```python
from build123d import *

# Parameters (mm, degrees)
ESQUISSE1_R                                   = 7
BOSS_EXTRU_1_DEPTH                            = 60
ESQUISSE3_R                                   = 7.5
BOSS_EXTRU_2_DEPTH                            = 62
ESQUISSE4_R                                   = 7.5
BOSS_EXTRU_3_DEPTH                            = 12
ESQUISSE5_R                                   = 7
BOSS_EXTRU_4_DEPTH                            = 26
ENL_V_MAT_EXTRU_1_DEPTH                       = 2.96
ENL_V_MAT_EXTRU_2_DEPTH                       = 2.96
TROU_POUR_TARAUDAGE_POUR_TROU_TARAUD_M6_D     = 5
TROU_POUR_TARAUDAGE_POUR_TROU_TARAUD_M6_DEPTH = 15
TROU_POUR_TARAUDAGE_POUR_TROU_TARAUD_M6_TIP   = 1.502151548
TROU_POUR_TARAUDAGE_POUR_TROU_TARAUD_2_D      = 5
TROU_POUR_TARAUDAGE_POUR_TROU_TARAUD_2_DEPTH  = 15
TROU_POUR_TARAUDAGE_POUR_TROU_TARAUD_2_TIP    = 1.502151548


with BuildPart() as part:
    # Esquisse1 → Boss.-Extru.1 (new body)
    with BuildSketch(Plane.XY):
        Circle(ESQUISSE1_R)
    extrude(amount=BOSS_EXTRU_1_DEPTH)

    # Esquisse3 → Boss.-Extru.2 (add)
    with BuildSketch(Plane.XY.offset(60)):
        Circle(ESQUISSE3_R)
    extrude(amount=BOSS_EXTRU_2_DEPTH)

    # Esquisse4 → Boss.-Extru.3 (add)
    with BuildSketch(Plane.XY.offset(122)):
        Circle(ESQUISSE4_R)
    extrude(amount=BOSS_EXTRU_3_DEPTH)

    # Esquisse5 → Boss.-Extru.4 (add)
    with BuildSketch(Plane.XY.offset(134)):
        Circle(ESQUISSE5_R)
    extrude(amount=BOSS_EXTRU_4_DEPTH)

    # Esquisse7 → Enlèv. mat.-Extru.1 (cut)
    with BuildSketch(Plane(origin=(7, 0, 0), x_dir=(0, 0, -1), z_dir=(1, 0, 0))):
        with BuildLine():
            Line((-155, 2.5), (-139, 2.5))
            ThreePointArc((-139, 2.5), (-136.5, 0), (-139, -2.5))
            Line((-139, -2.5), (-155, -2.5))
            ThreePointArc((-155, -2.5), (-157.5, 0), (-155, 2.5))
        make_face()
    extrude(amount=-ENL_V_MAT_EXTRU_1_DEPTH, mode=Mode.SUBTRACT)

    # Esquisse8 → Enlèv. mat.-Extru.2 (cut)
    with BuildSketch(Plane(origin=(7, 0, 0), x_dir=(0, 0, -1), z_dir=(1, 0, 0))):
        with BuildLine():
            Line((-10, -2.5), (-50, -2.5))
            ThreePointArc((-50, -2.5), (-52.5, 0), (-50, 2.5))
            Line((-50, 2.5), (-10, 2.5))
            ThreePointArc((-10, 2.5), (-7.5, 0), (-10, -2.5))
        make_face()
    extrude(amount=-ENL_V_MAT_EXTRU_2_DEPTH, mode=Mode.SUBTRACT)

    # Trou pour taraudage pour trou taraud_ M6
    with Locations(Plane(origin=(0, 0, 0), x_dir=(-1, 0, 0), z_dir=(0, 0, -1))):
        with Locations((0, 0)):
            Hole(TROU_POUR_TARAUDAGE_POUR_TROU_TARAUD_M6_D / 2, depth=TROU_POUR_TARAUDAGE_POUR_TROU_TARAUD_M6_DEPTH)
            with Locations((0, 0, -(TROU_POUR_TARAUDAGE_POUR_TROU_TARAUD_M6_DEPTH + TROU_POUR_TARAUDAGE_POUR_TROU_TARAUD_M6_TIP / 2))):  # 118° drill point
                Cone(0, TROU_POUR_TARAUDAGE_POUR_TROU_TARAUD_M6_D / 2, TROU_POUR_TARAUDAGE_POUR_TROU_TARAUD_M6_TIP, mode=Mode.SUBTRACT)

    # Trou pour taraudage pour trou taraud 2
    with Locations(Plane.XY.offset(160)):
        with Locations((0, 0)):
            Hole(TROU_POUR_TARAUDAGE_POUR_TROU_TARAUD_2_D / 2, depth=TROU_POUR_TARAUDAGE_POUR_TROU_TARAUD_2_DEPTH)
            with Locations((0, 0, -(TROU_POUR_TARAUDAGE_POUR_TROU_TARAUD_2_DEPTH + TROU_POUR_TARAUDAGE_POUR_TROU_TARAUD_2_TIP / 2))):  # 118° drill point
                Cone(0, TROU_POUR_TARAUDAGE_POUR_TROU_TARAUD_2_D / 2, TROU_POUR_TARAUDAGE_POUR_TROU_TARAUD_2_TIP, mode=Mode.SUBTRACT)


solid = part.part
```
For this review, take the finished solid that the model builds, in its own axes (mm). A direction names the side the tool comes from. Coordinates: 2 decimals unless noted, no trailing zeros. Order: outer loops, then holes, each group sorted by start corner. A loop starts at its lowest first (then second) coordinate and runs counter-clockwise, first axis right, second up. Notation, with made-up numbers: (52, 28) -> (59, 28) arc R23 cw to (59, 55) -> close; hole circle Ø1 at (76.5, 21). An arc over 180 degrees is marked (long way). Answer as CSV lines item,"result".
Q1. We need section C-C (x = -4.5). State the section outline as (y, z) points, plus the area to 3 significant figures.
Model answer:
outline,"(-6, 60) -> (-5.36, 60) -> (-5.36, 0) -> (5.36, 0) -> (5.36, 60) -> (6, 60) -> (6, 134) -> (5.36, 134) -> (5.36, 160) -> (-5.36, 160) -> (-5.36, 134) -> (-6, 134) -> close"
area,"1,810 mm2"
Q2. We need section B-B (z = 55.5). State the section outline as (x, y) points, plus the area to 3 significant figures.
Model answer:
outline,"circle Ø14 at (0, 0)"
area,"154 mm2"
Q3. We need section A-A (y = 4). State the section outline as (x, z) points, plus the area to 3 significant figures.
Model answer:
outline,"(-6.34, 60) -> (-5.74, 60) -> (-5.74, 0) -> (5.74, 0) -> (5.74, 60) -> (6.34, 60) -> (6.34, 134) -> (5.74, 134) -> (5.74, 160) -> (-5.74, 160) -> (-5.74, 134) -> (-6.34, 134) -> close"
area,"1,930 mm2"
Q4. Clearance check with flat-ended pins moving along their axes: pin 1 Ø8 at (x, y) = (0, 0) entering from -Z; pin 2 Ø1.2 at (x, z) = (5, 25.5) entering from +Y; pin 3 Ø2 at (x, z) = (5, 150) entering from -Y; pin 4 Ø5.5 at (y, z) = (0.5, 23.5) entering from +X. State where each tip first meets the part, or that it passes through.
Model answer:
pin 1,"stops at z = 0"
pin 2,"stops at y = 5.44"
pin 3,"stops at y = -5.74"
pin 4,"stops at x = 6.54"
Q5. We need section D-D (z = 76). State the section outline as (x, y) points.
Model answer:
outline,"circle Ø15 at (0, 0)"
Q6. Wall thickness on line 1 along Y through (x, z) = (0, 9.5); line 2 along X through (y, z) = (-0.25, 112); line 3 along Y through (x, z) = (6, 27.5): over which ranges is each line inside the solid? List them lowest first. Write a range as [from, to].
Model answer:
line 1,"y = [-7, -2.5], [2.5, 7]"
line 2,"x = [-7.5, 7.5]"
line 3,"y = [-3.61, -2.5], [2.5, 3.61]"
Q7. Draft analysis for pull direction Z (two halves, no side actions). For faces 5 (the face through (0, -3, 0)), 6 (the face through (5.5, 0.1, 136.5)), 7 (the face through (7, 2, 134)), 8 (the face through (-7.493, 0.33, 96.482)), state which applies: released by +Z, released by -Z, zero draft, split by the parting line, or undercut.
Model answer:
face 5,"released by -Z"
face 6,"undercut"
face 7,"released by +Z"
face 8,"zero draft"
Q8. For faces 1 (the face through (0.54, -2.44, 152.4)), 2 (the face through (5, -2.5, 30)), 3 (the face through (-0.54, -2.44, 7.6)), 4 (the face through (0, -3, 160)), list the 3-axis set-ups (+Z, -Z, +X, -X, +Y, -Y) from which the entire face can be reached by the end or side of a thin tool; tool diameter is ignored.
Model answer:
face 1,"+Z"
face 2,"+X"
face 3,"-Z"
face 4,"+Z, +X, -X, +Y, -Y"
